The listing builds one solid part. Answer for the finished solid, in the listing's coordinates (mm). A direction names the side the tool comes from. Coordinates: 2 decimals unless noted, no trailing zeros. Order: outer loops, then holes, each group sorted by start corner. A loop starts at its lowest first (then second) coordinate and runs counter-clockwise, first axis right, second up. Notation, with made-up numbers: (11.5, 45.25) -> (58.5, 45.25) arc R26 cw to (58.5, 83.25) -> close; hole circle Ø10 at (-10, -29.75). An arc over 180 degrees is marked (long way). Write item = value, one per line.
from build123d import *

# Parameters (mm, degrees)
SKETCH_RADAR_SEAT_W             = 65
SKETCH_RADAR_SEAT_H             = 68
RADAR_SEAT_DEPTH                = 4
LATERAL_STOPS_START             = 4
SKETCH_LATERAL_STOPS_W          = 3
SKETCH_LATERAL_STOPS_H          = 31
LATERAL_STOPS_DEPTH             = 9
POST_M3_START                   = -1
SKETCH_POST_M3_R                = 1.7
POST_M3_DEPTH                   = 7
TOP_SCREW_HEAD_RELIEFS_START    = 4
SKETCH_TOP_SCREW_HEAD_RELIEFS_R = 3.2
TOP_SCREW_HEAD_RELIEFS_DEPTH    = 3.7
RETENTION_STRAP_SLOTS_START     = -1
SKETCH_RETENTION_STRAP_SLOTS_W  = 3
SKETCH_RETENTION_STRAP_SLOTS_H  = 12
RETENTION_STRAP_SLOTS_DEPTH     = 7


with BuildPart() as part:
    # Sketch_Radar_seat → Radar_seat (new body)
    with BuildSketch(Plane.XY):
        with Locations((0, -9)):
            Rectangle(SKETCH_RADAR_SEAT_W, SKETCH_RADAR_SEAT_H)
    extrude(amount=RADAR_SEAT_DEPTH)

    # Sketch_Lateral_stops → Lateral_stops (add)
    with BuildSketch(Plane.XY.offset(LATERAL_STOPS_START)):
        with Locations((-21.4, 0)):
            Rectangle(SKETCH_LATERAL_STOPS_W, SKETCH_LATERAL_STOPS_H)
        with Locations((21.4, 0)):
            Rectangle(SKETCH_LATERAL_STOPS_W, SKETCH_LATERAL_STOPS_H)
    extrude(amount=LATERAL_STOPS_DEPTH)

    # Sketch_Post_M3 → Post_M3 (cut)
    with BuildSketch(Plane.XY.offset(POST_M3_START)):
        with Locations((-25, -37)):
            Circle(SKETCH_POST_M3_R)
        with Locations((-25, -9)):
            Circle(SKETCH_POST_M3_R)
        with Locations((25, -37)):
            Circle(SKETCH_POST_M3_R)
        with Locations((25, -9)):
            Circle(SKETCH_POST_M3_R)
    extrude(amount=POST_M3_DEPTH, mode=Mode.SUBTRACT)

    # Sketch_Top_screw_head_reliefs → Top_screw_head_reliefs (cut)
    with BuildSketch(Plane.XY.offset(TOP_SCREW_HEAD_RELIEFS_START)):
        with Locations((-25, -9)):
            Circle(SKETCH_TOP_SCREW_HEAD_RELIEFS_R)
        with Locations((25, -9)):
            Circle(SKETCH_TOP_SCREW_HEAD_RELIEFS_R)
    extrude(amount=TOP_SCREW_HEAD_RELIEFS_DEPTH, mode=Mode.SUBTRACT)

    # Sketch_Retention_strap_slots → Retention_strap_slots (cut)
    with BuildSketch(Plane.XY.offset(RETENTION_STRAP_SLOTS_START)):
        with Locations((-25, 0)):
            Rectangle(SKETCH_RETENTION_STRAP_SLOTS_W, SKETCH_RETENTION_STRAP_SLOTS_H)
        with Locations((25, 0)):
            Rectangle(SKETCH_RETENTION_STRAP_SLOTS_W, SKETCH_RETENTION_STRAP_SLOTS_H)
    extrude(amount=RETENTION_STRAP_SLOTS_DEPTH, mode=Mode.SUBTRACT)


solid = part.part
Q1. Section C-C, the plane y = -9 is taken. Give the vertices of the cut face in (x, z).
The answers:
outline = (-32.5, 0) -> (-26.7, 0) -> (-26.7, 4) -> (-32.5, 4) -> close; (-23.3, 0) -> (23.3, 0) -> (23.3, 4) -> (21.8, 4) -> (21.8, 7.7) -> (22.9, 7.7) -> (22.9, 13) -> (19.9, 13) -> (19.9, 4) -> (-19.9, 4) -> (-19.9, 13) -> (-22.9, 13) -> (-22.9, 7.7) -> (-21.8, 7.7) -> (-21.8, 4) -> (-23.3, 4) -> close; (26.7, 0) -> (32.5, 0) -> (32.5, 4) -> (26.7, 4) -> close
Q2. Section B-B, the plane x = 25 is taken. Give the vertices of the cut face in (y, z), plus the area to 3 significant figures.
The answers:
outline = (-43, 0) -> (-38.7, 0) -> (-38.7, 4) -> (-43, 4) -> close; (-35.3, 0) -> (-10.7, 0) -> (-10.7, 4) -> (-35.3, 4) -> close; (-7.3, 0) -> (-6, 0) -> (-6, 4) -> (-7.3, 4) -> close; (6, 0) -> (25, 0) -> (25, 4) -> (6, 4) -> close
area = 197 mm2
Q3. Each of these flat-tipped pins is pushed along its axis until it touches: pin 1 Ø1.2 at (x, y) = (22, -8) entering from -Z; pin 2 Ø4.5 at (y, z) = (-1, 7.5) entering from -X; pin 3 Ø6 at (x, y) = (-20, -22) entering from +Z; pin 4 Ø2.5 at (y, z) = (3, 6.5) entering from +X. Where does it stop, or does it pass through?
The answers:
pin_1 = 0
pin_2 = -22.9
pin_3 = 4
pin_4 = 22.9
Q4. Find the intervals of material crossed by line 1 along Y through (x, z) = (25, 0.9); line 2 along X through (y, z) = (-37, 2.4); line 3 along X through (y, z) = (-2, 8.5), in increasing order.
The answers:
line_1 = -43 to -38.7, -35.3 to -10.7, -7.3 to -6, 6 to 25
line_2 = -32.5 to -26.7, -23.3 to 23.3, 26.7 to 32.5
line_3 = -22.9 to -19.9, 19.9 to 22.9
Q5. Section A-A, the plane z = 6 is taken. Give the vertices of the cut face in (x, y), plus the area to 3 significant figures.
The answers:
outline = (-22.9, -15.5) -> (-19.9, -15.5) -> (-19.9, 15.5) -> (-22.9, 15.5) -> (-22.9, -6.59) arc R3.2 cw to (-22.9, -11.41) -> close; (19.9, -15.5) -> (22.9, -15.5) -> (22.9, -11.41) arc R3.2 cw to (22.9, -6.59) -> (22.9, 15.5) -> (19.9, 15.5) -> close
area = 179 mm2
Q6. A tool of negligible diameter and unlimited length cuts with its end or side. For faces 4 (the face through (25, -6, 2)), 5 (the face through (-21, 15.5, 8)), 6 (the face through (-22.9, 0, 8)), from which of +Z, -Z, +X, -X, +Y, -Y can it reach the whole face along a straight path? Write none if from no direction.
The answers:
face_4 = +Z, -Z
face_5 = +Z, +X, -X, +Y
face_6 = +Z, -X, +Y, -Y
Q7. The mould has two halves that part along Z. Classify faces 1 (the face through (21.8, -9, 5.8)), 2 (the face through (21, 15.5, 8)), 3 (the face through (21, 0, 13)): released by +Z, released by -Z, zero draft, split by the parting line, or undercut.
The answers:
face_1 = undercut
face_2 = zero draft
face_3 = released by +Z
Q8. Section D-D, the plane z = 2.25 is taken. Give the vertices of the cut face in (x, y), plus the area to 3 significant figures.
The answers:
outline = (-32.5, -43) -> (32.5, -43) -> (32.5, 25) -> (-32.5, 25) -> close; hole circle Ø3.4 at (-25, -37); hole circle Ø3.4 at (-25, -9); hole (-26.5, -6) -> (-23.5, -6) -> (-23.5, 6) -> (-26.5, 6) -> close; hole circle Ø3.4 at (25, -37); hole circle Ø3.4 at (25, -9); hole (23.5, -6) -> (26.5, -6) -> (26.5, 6) -> (23.5, 6) -> close
area = 4,310 mm2
